Model file for the job. Use its own axes, mm. Round coordinates to 2 decimals unless told otherwise and drop trailing zeros. Order: outer loops, then holes, each group sorted by start corner. A loop starts at its lowest first (then second) coordinate and runs counter-clockwise, first axis right, second up. Notation, with made-up numbers: (86, 25) - (144, 25) arc R16 ccw to (144, 40) - close; hole circle Ø9 at (31, -2.75). An arc over 180 degrees is marked (long way). Write item = value, one per line.
```python
from build123d import *

# Parameters (mm, degrees)
BOSS_EXTRUDE1_DEPTH      = 2.6
BOSS_EXTRUDE1_DEPTH_BACK = 2.6
SKETCH2_R                = 3
SKETCH3_OUTSIDE_W        = 50.698
SKETCH3_OUTSIDE_H        = 52.246
SKETCH3_OUTSIDE_R        = 5
CUT_EXTRUDE1_DEPTH       = 10.239769117
CUT_EXTRUDE1_DRAFT       = -60
MIRROR1_COPY_1_SKETCH_W  = 50.698
MIRROR1_COPY_1_SKETCH_H  = 52.246
MIRROR1_COPY_1_SKETCH_R  = 5
MIRROR1_COPY_1_DEPTH     = 10.239769117
MIRROR1_COPY_1_DRAFT     = -60


with BuildPart() as part:
    # Sketch2 → Boss-Extrude1 (new, two sides: drawn at the far end of the back side and taken through both)
    with BuildSketch(Plane.XY.offset(-BOSS_EXTRUDE1_DEPTH_BACK)):
        Polygon((0, 5.773502692), (-5, 2.886751346), (-5, -2.886751346), (0, -5.773502692), (5, -2.886751346), (5, 2.886751346), align=None)
        Circle(SKETCH2_R, mode=Mode.SUBTRACT)
    extrude(amount=BOSS_EXTRUDE1_DEPTH + BOSS_EXTRUDE1_DEPTH_BACK)


with BuildPart() as cut_extrude1_tool:
    # Sketch3 outside → Cut-Extrude1 (with draft: the straight prism first)
    with BuildSketch(Plane.XY.offset(2.6)):
        Rectangle(SKETCH3_OUTSIDE_W, SKETCH3_OUTSIDE_H)
        Circle(SKETCH3_OUTSIDE_R, mode=Mode.SUBTRACT)
    extrude(amount=-CUT_EXTRUDE1_DEPTH)
    # Cut-Extrude1: the draft: its side faces are tilted about the plane it starts from
    cut_extrude1_sides = [cut_extrude1_tool.faces().sort_by_distance(p)[0] for p in [
        (0, -26.123, -2.519884558),
        (25.349, 0, -2.519884558),
        (0, 26.123, -2.519884558),
        (-25.349, 0, -2.519884558),
        (-5, 0, -2.519884558),
    ]]
    draft(cut_extrude1_sides, Plane.XY.offset(2.6), CUT_EXTRUDE1_DRAFT)


with BuildPart() as part_1:
    add(part.part)

    # Cut-Extrude1: cut by cut_extrude1_tool
    add(cut_extrude1_tool.part, mode=Mode.SUBTRACT)


with BuildPart() as mirror1_copy_1_tool:
    # Mirror1 copy 1 sketch → Mirror1 copy 1 (with draft: the straight prism first)
    with BuildSketch(Plane(origin=(0, 0, -2.6), x_dir=(1, 0, 0), z_dir=(0, 0, -1))):
        Rectangle(MIRROR1_COPY_1_SKETCH_W, MIRROR1_COPY_1_SKETCH_H)
        Circle(MIRROR1_COPY_1_SKETCH_R, mode=Mode.SUBTRACT)
    extrude(amount=-MIRROR1_COPY_1_DEPTH)
    # Mirror1 copy 1: the draft: its side faces are tilted about the plane it starts from
    mirror1_copy_1_sides = [mirror1_copy_1_tool.faces().sort_by_distance(p)[0] for p in [
        (0, -26.123, 2.519884558),
        (25.349, 0, 2.519884558),
        (0, 26.123, 2.519884558),
        (-25.349, 0, 2.519884558),
        (-5, 0, 2.519884558),
    ]]
    draft(mirror1_copy_1_sides, Plane(origin=(0, 0, -2.6), x_dir=(1, 0, 0), z_dir=(0, 0, -1)), MIRROR1_COPY_1_DRAFT)


with BuildPart() as part_2:
    add(part_1.part)

    # Mirror1 copy 1: cut by mirror1_copy_1_tool
    add(mirror1_copy_1_tool.part, mode=Mode.SUBTRACT)


solid = part_2.part
```
1) Wall check: line 1 along Y through (x, z) = (-1.75, 1.45); line 2 along X through (y, z) = (1.75, -2.15); line 3 along X through (y, z) = (1.5, 0.65). Give the ranges that are in metal, low to high.
Conclusion:
line_1 = -4.76 to -2.44, 2.44 to 4.76
line_2 = -5 to -2.44, 2.44 to 5
line_3 = -5 to -2.6, 2.6 to 5
2) Cut at A-A (z = -1.45). Write the cut outline in (x, y), and give its area (3 significant figures).
Conclusion:
outline = (-5, -2.89) - (0, -5.77) - (5, -2.89) - (5, 2.89) - (0, 5.77) - (-5, 2.89) - close; hole circle Ø6 at (0, 0)
area = 58.3 mm^2
3) Flat gauge pins, fed straight in: pin 1 Ø1 at (x, z) = (1, 0) entering from +Y; pin 2 Ø1.5 at (x, z) = (1, 1.5) entering from -Y; pin 3 Ø1 at (x, z) = (-4, -1) entering from -Y. Where does each tip first touch, or does it go through?
Conclusion:
pin_1 = 5.48
pin_2 = -5.63
pin_3 = -3.75
4) Mould opens along Y. For faces 1 (the face through (3.3, 0.1, 2.6)), 2 (the face through (-3, 0, 0)), 3 (the face through (4.5, -2.58, -2.49)) say: +Y half, -Y half, draft (parallel to the pull), parting line (faces both ways), or undercut.
Conclusion:
face_1 = draft
face_2 = undercut
face_3 = -Y half
